For this review, use the dimensioned drawing (mm, ordinates from the lowest corner) and the shaded views. A direction names the side the tool comes from. Coordinates: 2 decimals unless noted, no trailing zeros. Write each loop counter-clockwise with the first axis right and the second up, starting at its lowest first coordinate (ties: lowest second). Pieces come first, ordered by that corner, then holes.
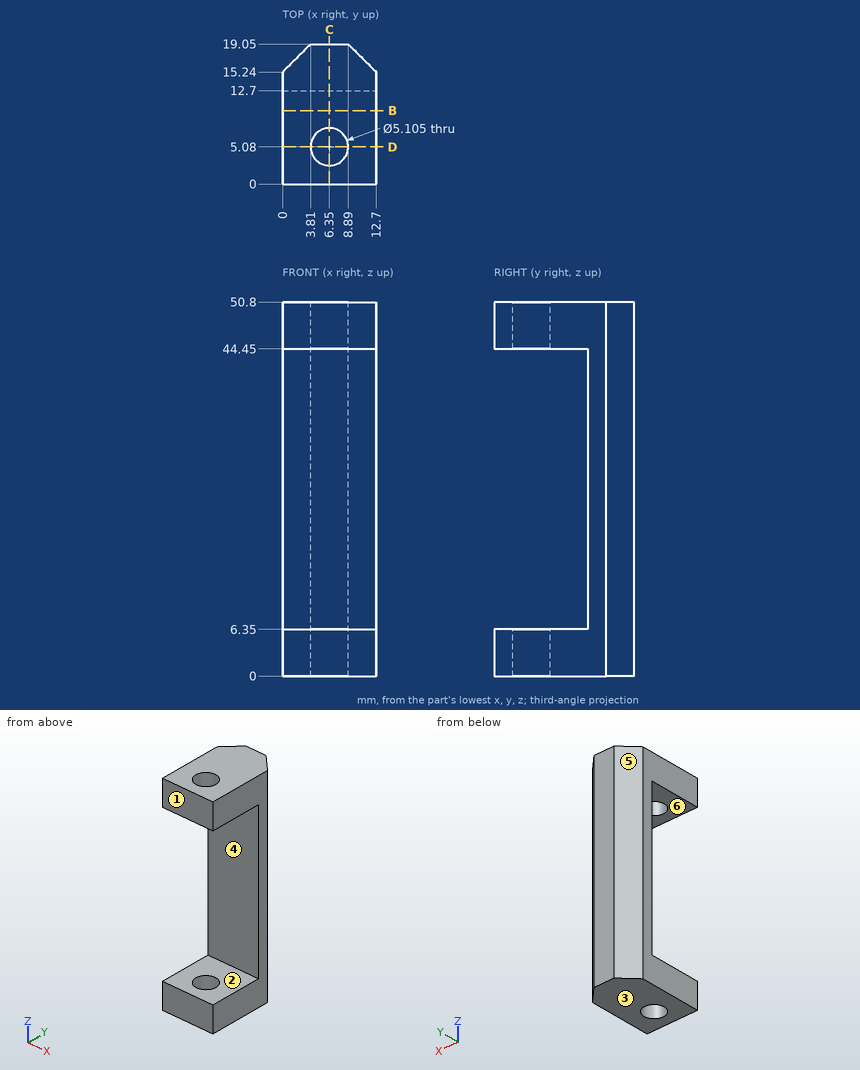
Item 1: For pin 1 (8 mm diameter, centred on y = 5.5, z = 15, fed in from -X); pin 2 (4 mm diameter, centred on x = 3.5, z = 27, fed in from -Y), all flat-tipped, find the tip position at first contact; note any pin that passes through.
Solved:
pin 1: passes through
pin 2: stops at y = 12.7
Item 2: Machinability: for the marked faces 5 and 6, which of the approach directions +Z, -Z, +X, -X, +Y, -Y give a long, thin tool a straight path to every point of the face, cutting with its end or side? Answer none if there is none.
Solved:
face 5: +Z, -Z, -X, +Y
face 6: +X, -X, -Y
Item 3: To check wall thickness, follow line 1 along Z through (x, y) = (2, 5.75); line 2 along Y through (x, z) = (6.35, 46.5). State the ranges of each line that lie inside material, in increasing order.
Solved:
line 1: z = 0 to 6.35, 44.45 to 50.8
line 2: y = 0 to 2.53, 7.63 to 19.05
Item 4: Take a section at C-C, the plane x = 6.35. Write out the cut boundary in (y, z), plus the area to 3 significant figures.
Solved:
outline: (0, 0) - (2.53, 0) - (2.53, 6.35) - (0, 6.35) - close; (0, 44.45) - (2.53, 44.45) - (2.53, 50.8) - (0, 50.8) - close; (7.63, 0) - (19.05, 0) - (19.05, 50.8) - (7.63, 50.8) - (7.63, 44.45) - (12.7, 44.45) - (12.7, 6.35) - (7.63, 6.35) - close
area: 419 mm2
Item 5: Take a section at B-B, the plane y = 10. Write out the cut boundary in (x, z), plus the area to 3 significant figures.
Solved:
outline: (0, 0) - (12.7, 0) - (12.7, 6.35) - (0, 6.35) - close; (0, 44.45) - (12.7, 44.45) - (12.7, 50.8) - (0, 50.8) - close
area: 161 mm2
Item 6: Take a section at D-D, the plane y = 5.08. Write out the cut boundary in (x, z).
Solved:
outline: (0, 0) - (3.8, 0) - (3.8, 6.35) - (0, 6.35) - close; (0, 44.45) - (3.8, 44.45) - (3.8, 50.8) - (0, 50.8) - close; (8.9, 0) - (12.7, 0) - (12.7, 6.35) - (8.9, 6.35) - close; (8.9, 44.45) - (12.7, 44.45) - (12.7, 50.8) - (8.9, 50.8) - close
Item 7: Mouldability with a two-part tool opening along Z and no side actions: class the marked faces 1, 2, 3 and 4 as pulls with the +Z half, pulls with the -Z half, needs draft (parallel to the pull), parting line crosses it, or undercut.
Solved:
face 1: needs draft
face 2: undercut
face 3: pulls with the -Z half
face 4: undercut
